Read the model definition and answer for the solid it produces. Units are mm, in the model's axes. A direction names the side the tool comes from. Coordinates: 2 decimals unless noted, no trailing zeros. Order: outer loops, then holes, each group sorted by start corner. A loop starts at its lowest first (then second) coordinate and runs counter-clockwise, first axis right, second up. Notation, with made-up numbers: M 59.5,28 L 67.5,28 A28 ccw 67.5,52 Z; hole C -8,-5 d8. An arc over 180 degrees is marked long. Use a Markdown table: item, result. Add a question column.
1) Each of these flat-tipped pins is pushed along its axis until it touches: pin 1 Ø8 at (x, y) = (-16, 24) entering from -Z; pin 2 Ø8 at (x, z) = (-5, -14) entering from +Y. Where does it stop, or does it pass through?
2) Find section C-C on z = -21.25. Write down the section's boundary in (x, y), plus the area to 3 significant figures.
3) The mould has two halves that part along Y. Classify faces 3 (the face through (18.95, 25.88, -2.28)), 4 (the face through (-22.5, 10, -4)), 5 (the face through (21.93, 33.4, -2.28)): released by +Y, released by -Y, zero draft, split by the parting line, or undercut.
4) Find section A-A on y = 24. Write down the section's boundary in (x, z), plus the area to 4 significant figures.
5) For faces 1 (the face through (0, 20, -4.5)), 2 (the face through (0, 34, -2)), determine the directions among +Z, -Z, +X, -X, +Y, -Y from which every point of the face is accessible in a straight line to the end or side of a thin tool.
6) Find the intervals of material crossed by probe 1 along X at (y, z) = (24, -2.6); probe 2 along X at (y, z) = (2.8, -15.75); probe 3 along Z at (x, y) = (-16.5, 3), in increasing order. Write a range as [from, to].
7) Find section B-B on z = -16. Write down the section's boundary in (x, y), plus the area to 3 significant figures.
8) Find section D-D on x = 6.5. Write down the section's boundary in (y, z), plus the area to 3 significant figures.
from build123d import *

# Parameters (mm, degrees)
CROQUIS1_R                   = 2.46
SALIENTE_EXTRUIR1_DEPTH      = 4.5
SALIENTE_EXTRUIR2_DEPTH      = 22.5
SALIENTE_EXTRUIR2_DEPTH_BACK = 22.5
CROQUIS2_W                   = 4.5
CROQUIS2_H                   = 34
CROQUIS3_R                   = 3.5
CORTAR_EXTRUIR1_DEPTH        = 22.5
REDONDEO1_R                  = 2
REDONDEO2_R                  = 2
REDONDEO3_R                  = 2


with BuildPart() as part:
    # Croquis1 → Saliente-Extruir1 (new body)
    with BuildSketch(Plane(origin=(0, 0, 0), x_dir=(1, 0, 0), z_dir=(0, 1, 0))):
        with BuildLine():
            Line((22.5, 0), (-22.5, 0))
            Line((-22.5, 0), (-22.5, 30))
            Line((-22.5, 30), (-14.866068747, 30))
            ThreePointArc((-14.866068747, 30), (0, 17), (14.866068747, 30))
            Line((14.866068747, 30), (22.5, 30))
            Line((22.5, 30), (22.5, 0))
        make_face()
        with Locations(Location((-16.25, 15.75, 0), (0, 0, 270))):
            Circle(CROQUIS1_R, mode=Mode.SUBTRACT)
        with Locations(Location((16.25, 15.75, 0), (0, 0, 90))):
            Circle(CROQUIS1_R, mode=Mode.SUBTRACT)
    extrude(amount=SALIENTE_EXTRUIR1_DEPTH)

    # Croquis2 → Saliente-Extruir2 (add, two sides: drawn at the far end of the back side and taken through both)
    with BuildSketch(Plane(origin=(0, 0, 0), x_dir=(0, 0, -1), z_dir=(1, 0, 0)).offset(-SALIENTE_EXTRUIR2_DEPTH_BACK)):
        with Locations((2.25, 17)):
            Rectangle(CROQUIS2_W, CROQUIS2_H)
    extrude(amount=SALIENTE_EXTRUIR2_DEPTH + SALIENTE_EXTRUIR2_DEPTH_BACK)

    # Croquis3 → Cortar-Extruir1 (cut)
    with BuildSketch(Plane(origin=(0, 0, -4.5), x_dir=(-1, 0, 0), z_dir=(0, 0, -1))):
        with Locations(Location((-16, 24, 0), (0, 0, 90))):
            Circle(CROQUIS3_R)
        with Locations(Location((16, 24, 0), (0, 0, 90))):
            Circle(CROQUIS3_R)
    extrude(amount=-CORTAR_EXTRUIR1_DEPTH, mode=Mode.SUBTRACT)

    # Redondeo1
    redondeo1_edges = [part.edges().sort_by_distance(p)[0] for p in [
        (0, 0, 0),
    ]]
    fillet(redondeo1_edges, radius=REDONDEO1_R)

    # Redondeo2
    redondeo2_edges = [part.edges().sort_by_distance(p)[0] for p in [
        (0, 4.5, -4.5),
    ]]
    fillet(redondeo2_edges, radius=REDONDEO2_R)

    # Redondeo3
    redondeo3_edges = [part.edges().sort_by_distance(p)[0] for p in [
        (-22.5, 34, -2.25),
        (22.5, 34, -2.25),
    ]]
    fillet(redondeo3_edges, radius=REDONDEO3_R)


solid = part.part
Check result:
| question | item | result |
|---|---|---|
| 1 | pin 1 | stops at z = -4.5 |
| 1 | pin 2 | stops at y = 4.5 |
| 2 | outline | M -22.5,0 L -10.46,0 L -10.46,4.5 L -22.5,4.5 Z; M 10.46,0 L 22.5,0 L 22.5,4.5 L 10.46,4.5 Z |
| 2 | area | 108 mm2 |
| 3 | face 3 | undercut |
| 3 | face 4 | zero draft |
| 3 | face 5 | released by +Y |
| 4 | outline | M -22.5,-4.5 L -19.5,-4.5 L -19.5,0 L -22.5,0 Z; M -12.5,-4.5 L 12.5,-4.5 L 12.5,0 L -12.5,0 Z; M 19.5,-4.5 L 22.5,-4.5 L 22.5,0 L 19.5,0 Z |
| 4 | area | 139.5 mm2 |
| 5 | face 1 | -Z, +X, -X, +Y |
| 5 | face 2 | +Z, -Z, +X, -X, +Y |
| 6 | probe 1 | x = [-22.5, -19.5], [-12.5, 12.5], [19.5, 22.5] |
| 6 | probe 2 | x = [-22.5, -18.71], [-13.79, 13.79], [18.71, 22.5] |
| 6 | probe 3 | z = [-30, -18.2], [-13.3, 0] |
| 7 | outline | M -22.5,0 L -18.7,0 L -18.7,4.5 L -22.5,4.5 Z; M -13.8,0 L 13.8,0 L 13.8,4.5 L -13.8,4.5 Z; M 18.7,0 L 22.5,0 L 22.5,4.5 L 18.7,4.5 Z |
| 7 | area | 158 mm2 |
| 8 | outline | M 0,-18.48 L 4.5,-18.48 L 4.5,-6.5 A2 cw 6.5,-4.5 L 34,-4.5 L 34,0 L 2,0 A2 ccw 0,-2 Z |
| 8 | area | 216 mm2 |
